Check sheet for the drawn part. Datum: minimum x, y, z corner. Units: mm. Give positions to 0.01 mm unless a question says otherwise; leave off trailing zeros. Loops run counter-clockwise (first coordinate to the right, second up) from the corner with the lowest first, then second, coordinate; pieces in that order, holes last. Notation, with made-up numbers: (45, -10) - (76, -10) arc R20 cw to (76, 20) - close; hole circle Ø11 at (53, 37.25). An arc over 180 degrees is marked (long way). Use a Markdown table: item, result. Add a question column.
1. Material ranges on L1, parallel to Z at x = 7.5, y = 1.3; L2, parallel to X at y = 0.5, z = 11.43; L3, parallel to X at y = 1.05, z = 3.81, recorded low to high.
2. Draft check along Z on the marked faces 1, 2 and 3. Enter one of: pulls with the +Z half, pulls with the -Z half, needs draft (parallel to the pull), parting line crosses it, or undercut.
3. Cross-section at B-B on y = 1.3. Enter the section's corners in (x, z), and give its area (3 significant figures).
4. Cross-section at C-C on x = 7. Enter the section's corners in (y, z).
5. Cross-section at D-D on x = 12.5. Enter the section's corners in (y, z), and give its area (3 significant figures).
6. Cross-section at A-A on z = 2. Enter the section's corners in (x, y).
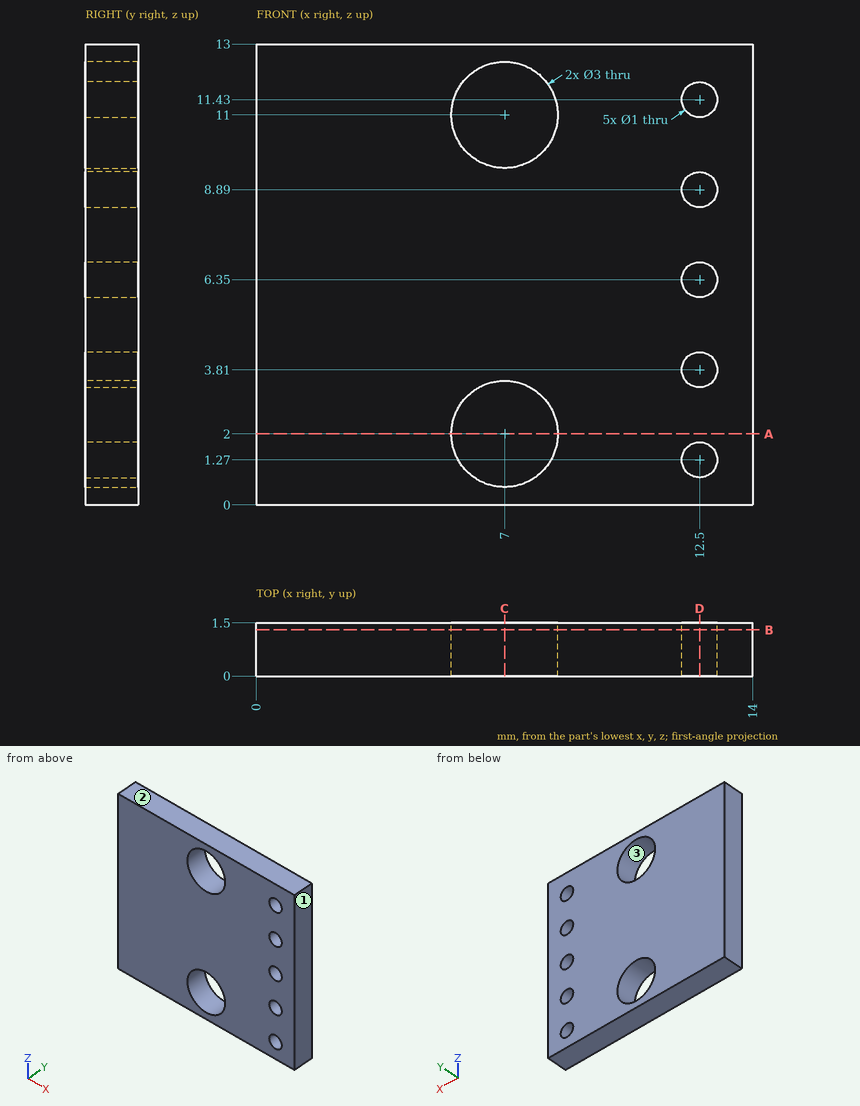
Values found:
| question | item | result |
|---|---|---|
| 1 | L1 | z = 0 to 0.59, 3.41 to 9.59, 12.41 to 13 |
| 1 | L2 | x = 0 to 5.56, 8.44 to 12, 13 to 14 |
| 1 | L3 | x = 0 to 12, 13 to 14 |
| 2 | face 1 | needs draft |
| 2 | face 2 | pulls with the +Z half |
| 2 | face 3 | undercut |
| 3 | outline | (0, 0) - (14, 0) - (14, 13) - (0, 13) - close; hole circle Ø3 at (7, 2); hole circle Ø3 at (7, 11); hole circle Ø1 at (12.5, 1.27); hole circle Ø1 at (12.5, 3.81); hole circle Ø1 at (12.5, 6.35); hole circle Ø1 at (12.5, 8.89); hole circle Ø1 at (12.5, 11.43) |
| 3 | area | 164 mm2 |
| 4 | outline | (0, 0) - (1.5, 0) - (1.5, 0.5) - (0, 0.5) - close; (0, 3.5) - (1.5, 3.5) - (1.5, 9.5) - (0, 9.5) - close; (0, 12.5) - (1.5, 12.5) - (1.5, 13) - (0, 13) - close |
| 5 | outline | (0, 0) - (1.5, 0) - (1.5, 0.77) - (0, 0.77) - close; (0, 1.77) - (1.5, 1.77) - (1.5, 3.31) - (0, 3.31) - close; (0, 4.31) - (1.5, 4.31) - (1.5, 5.85) - (0, 5.85) - close; (0, 6.85) - (1.5, 6.85) - (1.5, 8.39) - (0, 8.39) - close; (0, 9.39) - (1.5, 9.39) - (1.5, 10.93) - (0, 10.93) - close; (0, 11.93) - (1.5, 11.93) - (1.5, 13) - (0, 13) - close |
| 5 | area | 12.0 mm2 |
| 6 | outline | (0, 0) - (5.5, 0) - (5.5, 1.5) - (0, 1.5) - close; (8.5, 0) - (14, 0) - (14, 1.5) - (8.5, 1.5) - close |
